```python
from build123d import *

# Parameters (mm, degrees)
SKETCH1_W           = 13.843
SKETCH1_H           = 48.133
BOSS_EXTRUDE1_DEPTH = 4.7625
SKETCH2_R           = 3.3782
CUT_EXTRUDE1_DEPTH  = 5.7625
SKETCH3_W           = 13.843
SKETCH3_H           = 13.843
BOSS_EXTRUDE2_DEPTH = 14.31925
SKETCH6_W           = 13.843
SKETCH6_H           = 13.843
BOSS_EXTRUDE3_DEPTH = 19.812
SKETCH4_R           = 2.5527
CUT_EXTRUDE2_DEPTH  = 27.01925
SKETCH7_R           = 4.8641
CUT_EXTRUDE3_DEPTH  = 19.812
SKETCH8_W           = 13.843
SKETCH8_H           = 4.7625
BOSS_EXTRUDE4_DEPTH = 70.2818
SKETCH9_W           = 13.843
SKETCH9_H           = 13.843
BOSS_EXTRUDE5_DEPTH = 29.36875
SKETCH10_R          = 4.1275
CUT_EXTRUDE4_DEPTH  = 7.62
SKETCH11_R          = 2.2
CUT_EXTRUDE5_DEPTH  = 32.27375
SKETCH12_R          = 0.7493
BOSS_EXTRUDE6_DEPTH = 1.778


with BuildPart() as part:
    # Sketch1 → Boss-Extrude1 (new body)
    with BuildSketch(Plane.XY):
        with Locations((6.9215, 24.0665)):
            Rectangle(SKETCH1_W, SKETCH1_H)
    extrude(amount=BOSS_EXTRUDE1_DEPTH)

    # Sketch2 → Cut-Extrude1 (cut, through all)
    with BuildSketch(Plane(origin=(0, 0, 0), x_dir=(-1, 0, 0), z_dir=(0, 0, -1))):
        with Locations((-6.9215, 6.9215)):
            Circle(SKETCH2_R)
    extrude(amount=-CUT_EXTRUDE1_DEPTH, mode=Mode.SUBTRACT)

    # Sketch3 → Boss-Extrude2 (add)
    with BuildSketch(Plane.XY.offset(4.7625)):
        with Locations((6.9215, 41.2115)):
            Rectangle(SKETCH3_W, SKETCH3_H)
    extrude(amount=BOSS_EXTRUDE2_DEPTH)

    # Sketch6 → Boss-Extrude3 (add)
    with BuildSketch(Plane(origin=(0, 0, 0), x_dir=(-1, 0, 0), z_dir=(0, 0, -1))):
        with Locations((-6.9215, 41.2115)):
            Rectangle(SKETCH6_W, SKETCH6_H)
    extrude(amount=BOSS_EXTRUDE3_DEPTH)

    # Sketch4 → Cut-Extrude2 (cut)
    with BuildSketch(Plane(origin=(0, 0, 0), x_dir=(-1, 0, 0), z_dir=(0, 0, -1))):
        with Locations((-6.9215, 41.2115)):
            Circle(SKETCH4_R)
    extrude(amount=-CUT_EXTRUDE2_DEPTH, mode=Mode.SUBTRACT)

    # Sketch7 → Cut-Extrude3 (cut)
    with BuildSketch(Plane(origin=(0, 0, -19.812), x_dir=(-1, 0, 0), z_dir=(0, 0, -1))):
        with Locations((-6.9215, 41.2115)):
            Circle(SKETCH7_R)
    extrude(amount=-CUT_EXTRUDE3_DEPTH, mode=Mode.SUBTRACT)

    # Sketch8 → Boss-Extrude4 (add)
    with BuildSketch(Plane(origin=(0, 48.133, 0), x_dir=(1, 0, 0), z_dir=(0, 1, 0))):
        with Locations((6.9215, 17.43075)):
            Rectangle(SKETCH8_W, SKETCH8_H)
    extrude(amount=BOSS_EXTRUDE4_DEPTH)

    # Sketch9 → Boss-Extrude5 (add)
    with BuildSketch(Plane.XY.offset(-15.0495)):
        with Locations((6.9215, 111.4933)):
            Rectangle(SKETCH9_W, SKETCH9_H)
    extrude(amount=BOSS_EXTRUDE5_DEPTH)

    # Sketch10 → Cut-Extrude4 (cut)
    with BuildSketch(Plane(origin=(0, 0, -19.812), x_dir=(-1, 0, 0), z_dir=(0, 0, -1))):
        with Locations((-6.9215, 111.4933)):
            Circle(SKETCH10_R)
    extrude(amount=-CUT_EXTRUDE4_DEPTH, mode=Mode.SUBTRACT)

    # Sketch11 → Cut-Extrude5 (cut, through all)
    with BuildSketch(Plane(origin=(0, 0, -12.192), x_dir=(-1, 0, 0), z_dir=(0, 0, -1))):
        with Locations((-6.9215, 111.4933)):
            Circle(SKETCH11_R)
    extrude(amount=-CUT_EXTRUDE5_DEPTH, mode=Mode.SUBTRACT)

    # Sketch12 → Boss-Extrude6 (add)
    with BuildSketch(Plane(origin=(0, 48.133, 0), x_dir=(1, 0, 0), z_dir=(0, 1, 0))):
        with Locations((6.9215, -16.7005)):
            Circle(SKETCH12_R)
    extrude(amount=BOSS_EXTRUDE6_DEPTH)


solid = part.part
```
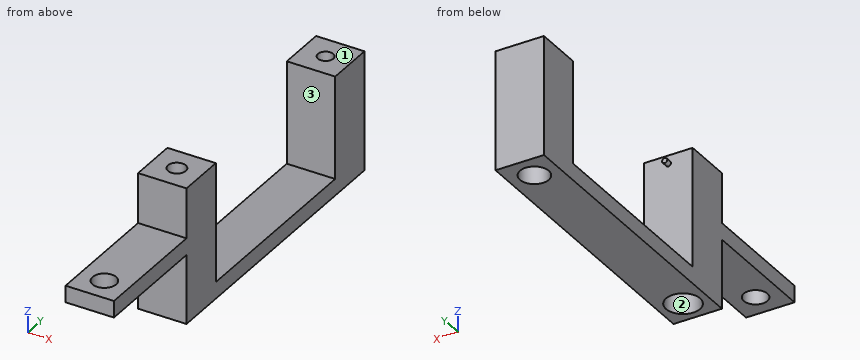
Geometry check sheet. Reference: the model listing, model coordinates, mm. Face numbers are marked on the shaded views. A direction names the side the tool comes from. Round coordinates to 2 decimals unless told otherwise and drop trailing zeros. Loops run counter-clockwise (first coordinate to the right, second up) from the corner with the lowest first, then second, coordinate; pieces in that order, holes last. Notation, with made-up numbers: (-10, 19) -> (25, 19) arc R19 ccw to (25, 24) -> close; hole circle Ø9 at (-6, -3.75). An arc over 180 degrees is marked (long way). Use a Markdown table: item, result.
(1) Set-up check for the marked faces 1, 2 and 3: record each of +Z, -Z, +X, -X, +Y, -Y from which the full face is reachable in a straight line by a thin tool's end or side.
Calculated:
| item | result |
|---|---|
| face 1 | +Z, +X, -X, +Y |
| face 2 | -Z |
| face 3 | +Z, +X, -X |
(2) Go/stop test with flat-tipped pins: P1, Ø4, axis at x = 6, y = 21, coming from the -Z side; P2, Ø4, axis at x = 12, y = 72.5, coming from the +Z side; P3, Ø0.7, axis at x = 7, z = 17, coming from the +Y side. Record where each tip stops, or that it passes through.
Calculated:
| item | result |
|---|---|
| P1 | z = 0 |
| P2 | z = -15.05 |
| P3 | y = 49.91 |
(3) Sectioned sample at A-A (z = -7). Enter the section's corners in (x, y), then the cut area to 3 significant figures.
Calculated:
| item | result |
|---|---|
| outline | (0, 34.29) -> (13.84, 34.29) -> (13.84, 48.13) -> (0, 48.13) -> close; (0, 104.57) -> (13.84, 104.57) -> (13.84, 118.41) -> (0, 118.41) -> close; hole circle Ø9.73 at (6.92, 41.21); hole circle Ø4.4 at (6.92, 111.49) |
| area | 294 mm² |
(4) Scan lines: probe 1 along Y at (x, z) = (7.25, -13); probe 2 along Y at (x, z) = (1.75, -13); probe 3 along Y at (x, z) = (3, 3). Record each from-to range of solid material in increasing order.
Calculated:
| item | result |
|---|---|
| probe 1 | 34.29 to 36.36, 46.06 to 48.13, 104.57 to 107.38, 115.61 to 118.41 |
| probe 2 | 34.29 to 48.13, 104.57 to 118.41 |
| probe 3 | 0 to 48.13, 104.57 to 118.41 |
(5) Sectioned sample at B-B (z = 7.5). Enter the section's corners in (x, y), then the cut area to 3 significant figures.
Calculated:
| item | result |
|---|---|
| outline | (0, 34.29) -> (13.84, 34.29) -> (13.84, 48.13) -> (0, 48.13) -> close; (0, 104.57) -> (13.84, 104.57) -> (13.84, 118.41) -> (0, 118.41) -> close; hole circle Ø5.11 at (6.92, 41.21); hole circle Ø4.4 at (6.92, 111.49) |
| area | 348 mm² |
(6) Sectioned sample at C-C (y = 52.5). Enter the section's corners in (x, z).
Calculated:
| item | result |
|---|---|
| outline | (0, -19.81) -> (13.84, -19.81) -> (13.84, -15.05) -> (0, -15.05) -> close |
